from build123d import *

# Parameters (mm, degrees)
F0_R     = 0.75
F0_R_2   = 0.53
F1_DEPTH = 1


# Not quite as in the source:
# - a feature names something its author has since deleted; it is built from what else it names


with BuildPart() as f1:
    # F0 (on Right) → F1 (new body)
    with BuildSketch(Plane.YZ):
        Polygon((8.384144865, 0), (0, 0), (0, -11.5), (11.5, -11.5), (11.5, 0), (11.2427603453, 0), (10.384144865, 0), (9.499944865, 0), align=None)
        with Locations((1.7500000088, -9.75)):
            Circle(F0_R, mode=Mode.SUBTRACT)
        with Locations((1.75, -7.75)):
            Circle(F0_R, mode=Mode.SUBTRACT)
        with Locations((3.7499851588, -10.5567658602)):
            Circle(F0_R_2, mode=Mode.SUBTRACT)
        with Locations((5.7499653617, -9.750009894)):
            Circle(F0_R, mode=Mode.SUBTRACT)
        with Locations((3.7499885936, -8.7499999912)):
            Circle(F0_R, mode=Mode.SUBTRACT)
        with Locations((3.7499923957, -6.75)):
            Circle(F0_R, mode=Mode.SUBTRACT)
        with Locations((5.7499752647, -7.7500098941)):
            Circle(F0_R, mode=Mode.SUBTRACT)
        with Locations((1.75, -5.75)):
            Circle(F0_R, mode=Mode.SUBTRACT)
        with Locations((1.75, -3.75)):
            Circle(F0_R, mode=Mode.SUBTRACT)
        with Locations((1.75, -1.75)):
            Circle(F0_R, mode=Mode.SUBTRACT)
        with Locations((3.7499961979, -4.75)):
            Circle(F0_R, mode=Mode.SUBTRACT)
        with Locations((5.7499851588, -5.7500098941)):
            Circle(F0_R, mode=Mode.SUBTRACT)
        with Locations((5.7499950529, -3.7500098941)):
            Circle(F0_R, mode=Mode.SUBTRACT)
        with Locations((3.75, -2.75)):
            Circle(F0_R, mode=Mode.SUBTRACT)
        with Locations((3.75, -0.94325)):
            Circle(F0_R_2, mode=Mode.SUBTRACT)
        with Locations((7.749955461, -10.5567658602)):
            Circle(F0_R_2, mode=Mode.SUBTRACT)
        with Locations((7.7499520262, -8.7500197836)):
            Circle(F0_R, mode=Mode.SUBTRACT)
        with Locations((7.7499680167, -6.7500197925)):
            Circle(F0_R, mode=Mode.SUBTRACT)
        with Locations((9.7499307145, -9.750039585)):
            Circle(F0_R, mode=Mode.SUBTRACT)
        with Locations((9.749950516, -7.7500395851)):
            Circle(F0_R, mode=Mode.SUBTRACT)
        with Locations((7.7499840072, -4.7500197926)):
            Circle(F0_R, mode=Mode.SUBTRACT)
        with Locations((5.750004947, -1.7500098941)):
            Circle(F0_R, mode=Mode.SUBTRACT)
        with Locations((7.7499999977, -2.7500197927)):
            Circle(F0_R, mode=Mode.SUBTRACT)
        with Locations((7.7499999977, -0.9432697927)):
            Circle(F0_R_2, mode=Mode.SUBTRACT)
        with Locations((9.7499703087, -5.7500395852)):
            Circle(F0_R, mode=Mode.SUBTRACT)
        with Locations((9.7499901013, -3.7500395853)):
            Circle(F0_R, mode=Mode.SUBTRACT)
        with Locations((9.750009894, -1.7500395854)):
            Circle(F0_R, mode=Mode.SUBTRACT)
        Polygon((9.499944865, 10), (9.499944865, 0), (10.384144865, 0), (11.2427603453, 0), (11.5, 0), (11.5, 10), (10.384144865, 10), align=None)
    extrude(amount=F1_DEPTH)


solid = f1.part
Read the model definition and answer for the solid it produces. Units are mm, in the model's axes. A direction names the side the tool comes from. Round coordinates to 2 decimals unless told otherwise and drop trailing zeros. Write each loop counter-clockwise with the first axis right and the second up, starting at its lowest first coordinate (ties: lowest second). Pieces come first, ordered by that corner, then holes. Notation, with made-up numbers: (66.25, -16.75) - (78.25, -16.75) arc R3 cw to (78.25, -12.75) - close; hole circle Ø5 at (-16.5, 79). An arc over 180 degrees is marked (long way). One line per question, with ' | ' between items. Start each with the question number.
1. This flat-tipped pin is pushed along its axis until it touches: pin 1 (1.4 mm diameter, centred on y = 3.75, z = -2.75, fed in from +X). Where does it stop, or does it pass through?
2. Find the intervals of material crossed by probe 1 along Z at (x, y) = (0.95, 5.75); probe 2 along Y at (x, z) = (0.5, -10.25); probe 3 along Z at (x, y) = (0.9, 6.25), in increasing order. Write a range as [from, to].
3. Section B-B (y = 1.75) is taken. Determine the outline of the cut face in (x, z), and give its area (3 significant figures).
4. Section A-A (y = 7.75) is taken. Determine the outline of the cut face in (x, z), and give its area (3 significant figures).
5. For faces 1 (the face through (0.5, 7, -6.7)), 2 (the face through (0.5, 4.8, 0)), determine the directions among +Z, -Z, +X, -X, +Y, -Y from which every point of the face is accessible in a straight line to the end or side of a thin tool.
6. Section D-D (z = 2.25) is taken. Determine the outline of the cut face in (x, y).
7. For a pull along Z with two mould halves and no side action, classify faces 3 (the face through (0.5, 9.5, 5.1)), 4 (the face through (0.5, 9, -3.7)), 5 (the face through (0.5, 10.5, 10)) as +Z half, -Z half, draft (parallel to the pull), parting line (faces both ways), or undercut.
8. Section C-C (x = 0.3) is taken. Give the number of separate pieces and of enclosed holes in the cut face, and give its area (3 significant figures).
Filled in:
1) pin 1: through
2) probe 1: [-11.5, -10.5], [-9, -8.5], [-7, -6.5], [-5, -4.5], [-3, -2.5], [-1, 0] | probe 2: [0, 1.19], [2.31, 3.32], [4.18, 5.19], [6.31, 7.32], [8.18, 9.19], [10.31, 11.5] | probe 3: [-11.5, -10.31], [-9.19, -8.31], [-7.19, -6.31], [-5.19, -4.31], [-3.19, -2.31], [-1.19, 0]
3) outline: (0, -11.5) - (1, -11.5) - (1, -10.5) - (0, -10.5) - close; (0, -9) - (1, -9) - (1, -8.5) - (0, -8.5) - close; (0, -7) - (1, -7) - (1, -6.5) - (0, -6.5) - close; (0, -5) - (1, -5) - (1, -4.5) - (0, -4.5) - close; (0, -3) - (1, -3) - (1, -2.5) - (0, -2.5) - close; (0, -1) - (1, -1) - (1, 0) - (0, 0) - close | area: 4.00 mm²
4) outline: (0, -11.5) - (1, -11.5) - (1, -11.09) - (0, -11.09) - close; (0, -10.03) - (1, -10.03) - (1, -9.5) - (0, -9.5) - close; (0, -8) - (1, -8) - (1, -7.5) - (0, -7.5) - close; (0, -6) - (1, -6) - (1, -5.5) - (0, -5.5) - close; (0, -4) - (1, -4) - (1, -3.5) - (0, -3.5) - close; (0, -2) - (1, -2) - (1, -1.47) - (0, -1.47) - close; (0, -0.41) - (1, -0.41) - (1, 0) - (0, 0) - close | area: 3.38 mm²
5) face 1: +X, -X | face 2: +Z, +X, -X, -Y
6) outline: (0, 9.5) - (1, 9.5) - (1, 11.5) - (0, 11.5) - close
7) face 3: draft | face 4: undercut | face 5: +Z half
8) separate pieces: 1 | enclosed holes: 27 | area: 108 mm²
